Verification items for the finished model (mm, model axes). Coordinates: 2 decimals unless noted, no trailing zeros. Write each loop counter-clockwise with the first axis right and the second up, starting at its lowest first coordinate (ties: lowest second). Pieces come first, ordered by that corner, then holes. Notation, with made-up numbers: (-24.75, 35) -> (-4.75, 35) arc R17 cw to (-4.75, 54) -> close; hole circle Ø3 at (41, 22). An arc over 180 degrees is marked (long way). Answer in a Markdown table with one row per item.
```python
from build123d import *

# Parameters (mm, degrees)
SKETCH1_W           = 25.4
SKETCH1_H           = 22.86
BOSS_EXTRUDE1_DEPTH = 5.715
CUT_EXTRUDE1_REACH  = 36.647


with BuildPart() as part:
    # Sketch1 → Boss-Extrude1 (new body)
    with BuildSketch(Plane.XY):
        with Locations((12.7, 11.43)):
            Rectangle(SKETCH1_W, SKETCH1_H)
    extrude(amount=BOSS_EXTRUDE1_DEPTH)

    # Sketch2 → Cut-Extrude1 (cut, up to next)
    with BuildSketch(Plane.XY.offset(5.715), mode=Mode.PRIVATE) as cut_extrude1_sk1:
        Polygon((5.15716279, 22.86), (25.4, 5.612386194), (25.4, 22.86), align=None)
    cut_extrude1_tool1 = extrude(cut_extrude1_sk1.sketch, amount=-CUT_EXTRUDE1_REACH, mode=Mode.PRIVATE) & part.part
    add(cut_extrude1_tool1.solids().sort_by_distance((18.652388, 17.110795, 5.715))[0], mode=Mode.SUBTRACT)


solid = part.part
```
1. Depth check by flat-ended pin: P1, Ø1.5, axis at x = 6.5, z = 1.5, coming from the +Y side. Enter the tip coordinate at first touch or a pass-through.
Geometry says:
| item | result |
|---|---|
| P1 | y = 22.35 |
2. Section check C-C, the plane y = 10. Record the boundary of the cut face in (x, z) (3 decimals).
Geometry says:
| item | result |
|---|---|
| outline | (0, 0) -> (20.25, 0) -> (20.25, 5.715) -> (0, 5.715) -> close |
3. Thickness scan on line 1 (Y direction, x = 23.75, z = 1.2); line 2 (Y direction, x = 6, z = 2.2); line 3 (X direction, y = 22.25, z = 3.6). Record the ranges inside material, lowest first. Write a range as from..to.
Geometry says:
| item | result |
|---|---|
| line 1 | 0..7.02 |
| line 2 | 0..22.14 |
| line 3 | 0..5.87 |
4. Section check A-A, the plane z = 1.45. Record the boundary of the cut face in (x, y).
Geometry says:
| item | result |
|---|---|
| outline | (0, 0) -> (25.4, 0) -> (25.4, 5.61) -> (5.16, 22.86) -> (0, 22.86) -> close |
5. Section check B-B, the plane x = 21.25. Record the boundary of the cut face in (y, z) (3 decimals).
Geometry says:
| item | result |
|---|---|
| outline | (0, 0) -> (9.148, 0) -> (9.148, 5.715) -> (0, 5.715) -> close |
